Part print with two shaded views. Sizes in mm from the minimum x, y, z corner. Give positions to 0.01 mm unless a question says otherwise; leave off trailing zeros. Order: outer loops, then holes, each group sorted by start corner. A loop starts at its lowest first (then second) coordinate and runs counter-clockwise, first axis right, second up. Notation, with made-up numbers: M 87,-15.5 L 134,-15.5 A21 cw 134,-6.5 Z; hole C -15,16 d1. An arc over 180 degrees is marked long. Answer as CSV lines item,"result".
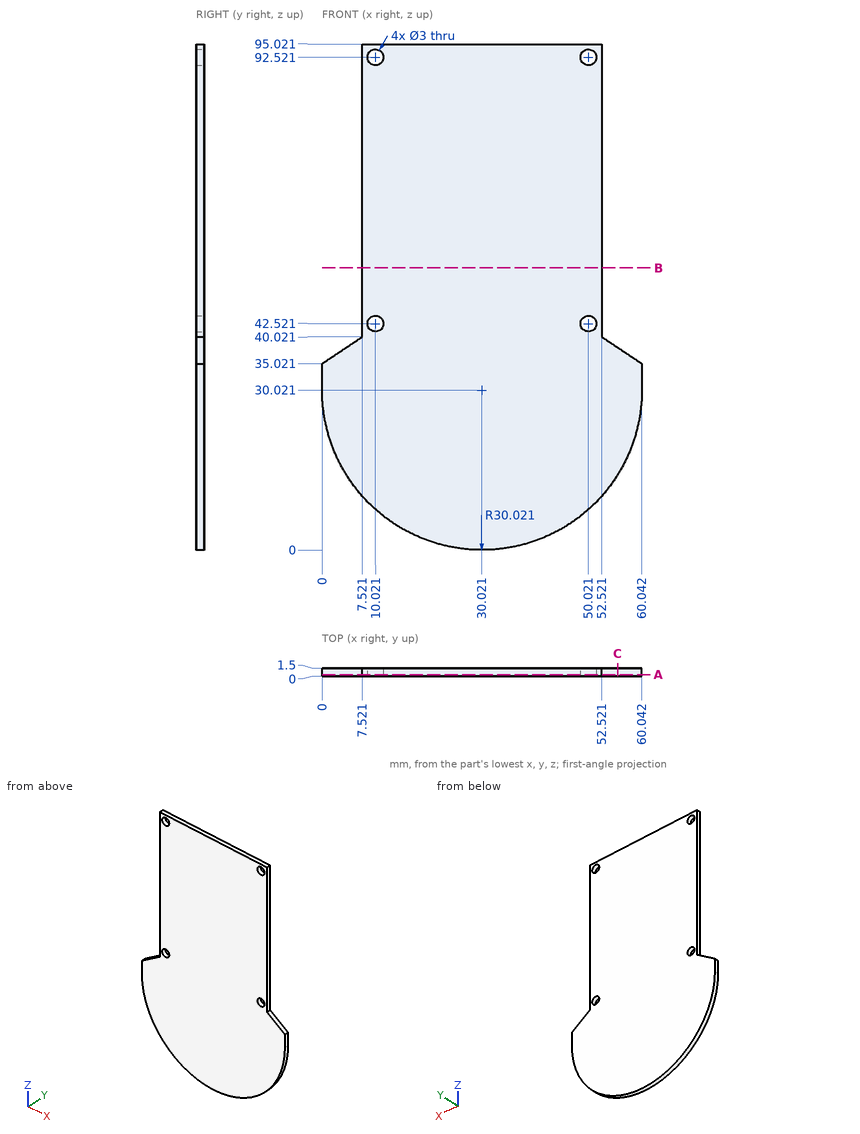
Item 1: Band-saw the part on C-C (x = 55.5). Give the cut face in (y, z), and give its area (3 significant figures).
Geometry says:
outline,"M 0,14.14 L 1.5,14.14 L 1.5,38.04 L 0,38.04 Z"
area,"35.8 mm2"
Item 2: Drop flat-ended pins along their axis: pin 1 (4 mm diameter, centred on x = 37, z = 38.5, fed in from -Y); pin 2 (0.8 mm diameter, centred on y = 1, z = 70, fed in from +X); pin 3 (1.8 mm diameter, centred on x = 50.02, z = 92.52, fed in from -Y). Give the stop position or say it passes through.
Geometry says:
pin 1,"stops at y = 0"
pin 2,"stops at x = 52.52"
pin 3,"passes through"
Item 3: Band-saw the part on B-B (z = 53). Give the cut face in (x, y).
Geometry says:
outline,"M 7.52,0 L 52.52,0 L 52.52,1.5 L 7.52,1.5 Z"
Item 4: Band-saw the part on A-A (y = 0.25). Give the cut face in (x, z).
Geometry says:
outline,"M 0,30.02 A30.02 ccw 60.04,30.02 L 60.04,35.02 L 52.52,40.02 L 52.52,95.02 L 7.52,95.02 L 7.52,40.02 L 0,35.02 Z; hole C 10.02,42.52 d3; hole C 10.02,92.52 d3; hole C 50.02,42.52 d3; hole C 50.02,92.52 d3"
Item 5: Probe line 1 along Z through (x, y) = (10, 0.1); line 2 along X through (y, z) = (0.5, 71); line 3 along X through (y, z) = (1, 38.5). List the from-to ranges inside material, lowest first. Write a range as from..to.
Geometry says:
line 1,"z = 7.65..41.02, 44.02..91.02, 94.02..95.02"
line 2,"x = 7.52..52.52"
line 3,"x = 5.23..54.81"
